```python
from build123d import *

# Parameters (mm, degrees)
BOSS_EXTRUDE1_DEPTH = 520
RIB15_REACH         = 866.242
SKETCH14_WALL_W     = 2151.777513516
SKETCH14_WALL_H     = 80


with BuildPart() as part:
    # Sketch1 → Boss-Extrude1 (new body)
    with BuildSketch(Plane.XY):
        with BuildLine():
            Line((-63.134983493, 0), (686.865016507, 0))
            Line((686.865016507, 0), (686.865016507, 60))
            Line((686.865016507, 60), (356.865016507, 60))
            Line((356.865016507, 60), (356.865016507, 230))
            ThreePointArc((356.865016507, 230), (489.699208945, 309.695349915), (541.865016507, 455.554871373))
            Line((541.865016507, 455.554871373), (461.865016507, 455.554871373))
            ThreePointArc((461.865016507, 455.554871373), (311.865016507, 305.554871373), (161.865016507, 455.554871373))
            Line((161.865016507, 455.554871373), (81.865016507, 455.554871373))
            ThreePointArc((81.865016507, 455.554871373), (134.03082407, 309.695349915), (266.865016507, 230))
            Line((266.865016507, 230), (266.865016507, 60))
            Line((266.865016507, 60), (-63.134983493, 60))
            Line((-63.134983493, 60), (-63.134983493, 0))
        make_face()
    extrude(amount=-BOSS_EXTRUDE1_DEPTH)

    # Sketch14 wall → Rib15 (add, up to next)
    with BuildSketch(Plane(origin=(9.365016507, 257.777435686, -260), x_dir=(-0.344177678967, -0.938904534711, 0), z_dir=(-0.938904534711, 0.344177678967, 0)), mode=Mode.PRIVATE) as rib15_sk1:
        Rectangle(SKETCH14_WALL_W, SKETCH14_WALL_H)
    rib15_tool1 = extrude(rib15_sk1.sketch, amount=-RIB15_REACH, mode=Mode.PRIVATE) - part.part
    add(rib15_tool1.solids().sort_by_distance((9.365016507, 257.777435686, -260))[0])


solid = part.part
```
Input: part model. Units: mm. Frame: model coordinates. A direction names the side the tool comes from. Round coordinates to 2 decimals unless told otherwise and drop trailing zeros. Loops run counter-clockwise (first coordinate to the right, second up) from the corner with the lowest first, then second, coordinate; pieces in that order, holes last. Notation, with made-up numbers: (59, -34) -> (83, -34) arc R37 cw to (83, 5) -> close; hole circle Ø3 at (72.25, 82.25). An arc over 180 degrees is marked (long way). One line per item, written item: value.
(1) Set-up query: faces 1 (the face through (132.64, 311.41, -408.46)), 2 (the face through (105, 176, -220)), 3 (the face through (502, 455.555, -256)), 4 (the face through (310, 178, -520)), 5 (the face through (356.865, 144, -256)). Return all of +Z, -Z, +X, -X, +Y, -Y with unobstructed straight access to the full face (end or side cutting, diameter ignored); none if empty.
Geometry check:
face 1: -Z, -X
face 2: +Z, -X
face 3: +Z, -Z, +X, -X, +Y
face 4: -Z, +X, -X, +Y, -Y
face 5: +Z, -Z, +X
(2) Section A-A (x = 518.5). Return the cut outline in (y, z), plus the area to 3 significant figures.
Geometry check:
outline: (0, -520) -> (60, -520) -> (60, 0) -> (0, 0) -> close; (354.55, -520) -> (455.55, -520) -> (455.55, 0) -> (354.55, 0) -> close
area: 83,700 mm2
(3) Section B-B (y = 395). Return the cut outline in (x, z), plus the area to 3 significant figures.
Geometry check:
outline: (59.67, -300) -> (89.98, -300) -> (89.98, -520) -> (174.63, -520) -> (174.63, 0) -> (89.98, 0) -> (89.98, -220) -> (59.67, -220) -> close; (449.1, -520) -> (533.75, -520) -> (533.75, 0) -> (449.1, 0) -> close
area: 90,500 mm2
(4) Pin query (flat end, axial travel): pin 1 (2 mm diameter, centred on x = 90, y = 75, fed in from -Z); pin 2 (8 mm diameter, centred on x = 44, z = -368, fed in from +Y); pin 3 (6 mm diameter, centred on x = 275, z = -258.5, fed in from +Y). Return the tip coordinate at first contact, or that it passes through.
Geometry check:
pin 1: z = -300
pin 2: y = 60
pin 3: y = 310.95
(5) Section D-D (y = 270.5). Return the cut outline in (x, z), plus the area to 3 significant figures.
Geometry check:
outline: (14.03, -300) -> (175.28, -300) -> (175.28, -520) -> (448.45, -520) -> (448.45, 0) -> (175.28, 0) -> (175.28, -220) -> (14.03, -220) -> close
area: 155,000 mm2
(6) Section C-C (z = -234.5). Return the cut outline in (x, y).
Geometry check:
outline: (-63.13, 0) -> (686.87, 0) -> (686.87, 60) -> (356.87, 60) -> (356.87, 230) arc R230 ccw to (541.87, 455.55) -> (461.87, 455.55) arc R150 cw to (161.87, 455.55) -> (81.87, 455.55) -> (-63.13, 60) -> close
(7) Mould query, pull axis Y, two halves, no side actions, for faces 6 (the face through (132.64, 311.41, -108.46)), 7 (the face through (307, 0, -256)), 8 (the face through (104, 60, -408)), 9 (the face through (310, 178, 0)). Classes: pulls with the +Y half, pulls with the -Y half, needs draft (parallel to the pull), parting line crosses it, or undercut.
Geometry check:
face 6: undercut
face 7: pulls with the -Y half
face 8: undercut
face 9: needs draft
(8) Material intervals for line 1 (X direction, y = 117, z = -93); line 2 (Z direction, x = 139, y = 80); line 3 (Y direction, x = 547, z = -453), sorted ascending. Write a range as [from, to].
Geometry check:
line 1: [266.87, 356.87]
line 2: [-300, -220]
line 3: [0, 60]
